Geometry check sheet. Reference: the model listing, model coordinates, mm. Round coordinates to 2 decimals unless told otherwise and drop trailing zeros. Write each loop counter-clockwise with the first axis right and the second up, starting at its lowest first coordinate (ties: lowest second). Pieces come first, ordered by that corner, then holes. Notation, with made-up numbers: (53.25, 76.25) -> (71.25, 76.25) arc R19 cw to (71.25, 83.25) -> close; hole circle Ø10 at (44.5, 20). An arc over 180 degrees is marked (long way). Return JSON: item names as keys, results as strings. Group by question number.
from build123d import *

# Parameters (mm, degrees)
SKETCH_1_W      = 600
SKETCH_1_H      = 480
SKETCH_1_R      = 11
SKETCH_1_R_2    = 2.75
SKETCH_1_R_3    = 13.5
EXTRUDE_1_DEPTH = 10
FILLET_1_R      = 20


with BuildPart() as part:
    # Sketch 1 → Extrude 1 (new body)
    with BuildSketch(Plane.XY):
        with Locations((-255, 0)):
            Rectangle(SKETCH_1_W, SKETCH_1_H)
        Circle(SKETCH_1_R, mode=Mode.SUBTRACT)
        with Locations((-17.67766953, 17.67766953)):
            Circle(SKETCH_1_R_2, mode=Mode.SUBTRACT)
        with Locations((17.67766953, 17.67766953)):
            Circle(SKETCH_1_R_2, mode=Mode.SUBTRACT)
        with Locations((-17.67766953, -17.67766953)):
            Circle(SKETCH_1_R_2, mode=Mode.SUBTRACT)
        with Locations((17.67766953, -17.67766953)):
            Circle(SKETCH_1_R_2, mode=Mode.SUBTRACT)
        with Locations((0, 185)):
            Circle(SKETCH_1_R_3, mode=Mode.SUBTRACT)
        with Locations((-17.67766953, 167.32233047)):
            Circle(SKETCH_1_R_2, mode=Mode.SUBTRACT)
        with Locations((17.67766953, 167.32233047)):
            Circle(SKETCH_1_R_2, mode=Mode.SUBTRACT)
        with Locations((17.67766953, 202.67766953)):
            Circle(SKETCH_1_R_2, mode=Mode.SUBTRACT)
        with Locations((-17.67766953, 202.67766953)):
            Circle(SKETCH_1_R_2, mode=Mode.SUBTRACT)
        with Locations((-17.67766953, -202.67766953)):
            Circle(SKETCH_1_R_2, mode=Mode.SUBTRACT)
        with Locations((17.67766953, -202.67766953)):
            Circle(SKETCH_1_R_2, mode=Mode.SUBTRACT)
        with Locations((17.67766953, -167.32233047)):
            Circle(SKETCH_1_R_2, mode=Mode.SUBTRACT)
        with Locations((-17.67766953, -167.32233047)):
            Circle(SKETCH_1_R_2, mode=Mode.SUBTRACT)
        with Locations((0, -185)):
            Circle(SKETCH_1_R_3, mode=Mode.SUBTRACT)
        with Locations((-535, 165)):
            Circle(SKETCH_1_R_2, mode=Mode.SUBTRACT)
        with Locations((-115, 165)):
            Circle(SKETCH_1_R_2, mode=Mode.SUBTRACT)
        with Locations((-115, -165)):
            Circle(SKETCH_1_R_2, mode=Mode.SUBTRACT)
        with Locations((-535, -165)):
            Circle(SKETCH_1_R_2, mode=Mode.SUBTRACT)
    extrude(amount=EXTRUDE_1_DEPTH)

    # Fillet 1
    fillet_1_edges = [part.edges().sort_by_distance(p)[0] for p in [
        (-555, -240, 5),
        (-555, 240, 5),
    ]]
    fillet(fillet_1_edges, radius=FILLET_1_R)


solid = part.part
1) Material ranges on probe 1 along Y at (x, z) = (0, 4.25); probe 2 along X at (y, z) = (200.5, 7); probe 3 along X at (y, z) = (165, 6), recorded low to high. Write a range as [from, to].
2) Sectioned sample at B-B on y = 185. Enter the section's corners in (x, z).
3) Go/stop test with a flat-tipped pin: P1, Ø8, axis at x = -472, y = 101, coming from the -Z side. Record where the tip stops, or that it passes through.
4) Sectioned sample at A-A on y = 0. Enter the section's corners in (x, z).
5) Mould release check, pull along Y, two halves, no side actions. Record for faces 1 (the face through (-9.95, 194.124, 4.93)), 2 (the face through (-259, 3, 10)), 3 (the face through (-549.297, 233.986, 5.07)), 4 (the face through (-2.93, -198.18, 4.93)): +Y half, -Y half, draft (parallel to the pull), parting line (faces both ways), or undercut.
Evaluation:
{
 "1": {"probe 1": "y = [-240, -198.5], [-171.5, -11], [11, 171.5], [198.5, 240]", "probe 2": "x = [-555, -19.36], [-16, 16], [19.36, 45]", "probe 3": "x = [-555, -537.75], [-532.25, -117.75], [-112.25, -19.15], [-16.2, 16.2], [19.15, 45]"},
 "2": {"outline": "(-555, 0) -> (-13.5, 0) -> (-13.5, 10) -> (-555, 10) -> close; (13.5, 0) -> (45, 0) -> (45, 10) -> (13.5, 10) -> close"},
 "3": {"P1": "stops at z = 0"},
 "4": {"outline": "(-555, 0) -> (-11, 0) -> (-11, 10) -> (-555, 10) -> close; (11, 0) -> (45, 0) -> (45, 10) -> (11, 10) -> close"},
 "5": {"face 1": "undercut", "face 2": "draft", "face 3": "+Y half", "face 4": "undercut"}
}
